Answer from the drawing. Dimensions are ordinates in mm from the lowest x, y and z of the part. Round coordinates to 2 decimals unless told otherwise and drop trailing zeros. Write each loop counter-clockwise with the first axis right and the second up, starting at its lowest first coordinate (ties: lowest second). Pieces come first, ordered by that corner, then holes. Notation, with made-up numbers: (4.25, -37) - (54.25, -37) arc R22 ccw to (54.25, -21) - close; hole circle Ø9 at (22.5, -28.75). An arc over 180 degrees is marked (long way). Answer as a JSON object with one key per item and string values.
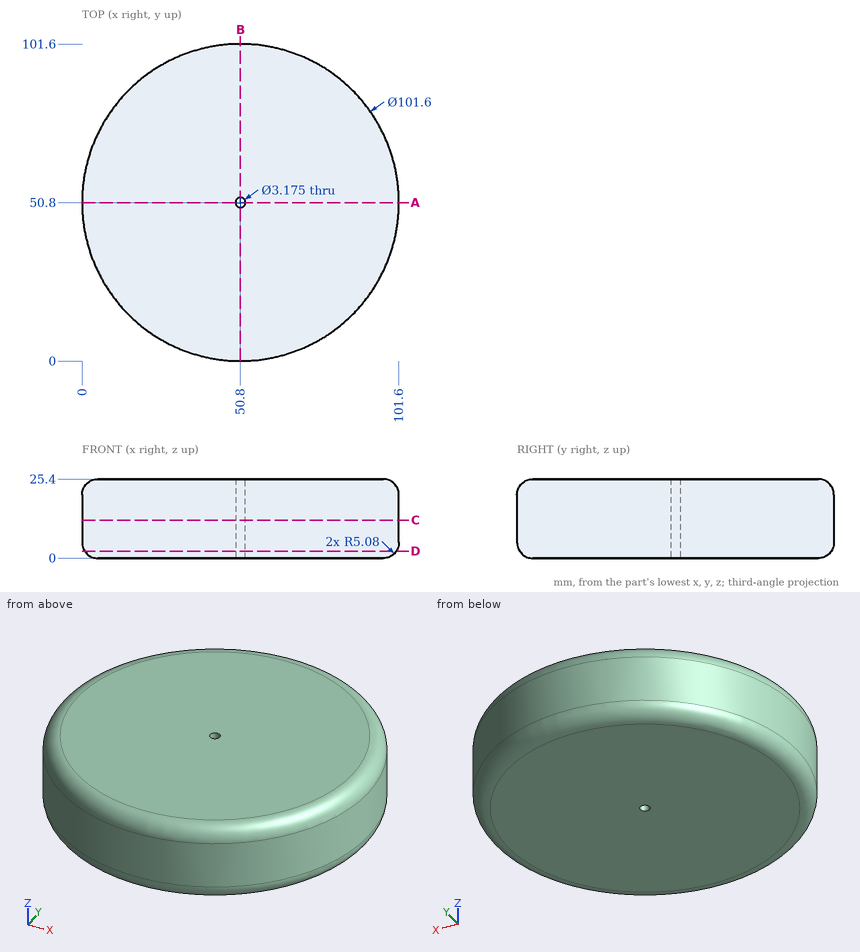
Item 1: A cutting plane is placed at D-D (z = 2.25). Write down the section's boundary in (x, y) (1 decimal), and give its area (3 significant figures).
Results found:
{"outline": "circle Ø99.9 at (50.8, 50.8); hole circle Ø3.2 at (50.8, 50.8)", "area": "7,830 mm²"}
Item 2: Each of these flat-tipped pins is pushed along its axis until it touches: P1, Ø10, axis at y = 21.5, z = 14.5, coming from the +X side; P2, Ø1, axis at x = 73, z = 12, coming from the +Y side; P3, Ø6, axis at x = 71, z = 14, coming from the +Y side; P4, Ø5, axis at x = 42.5, y = 91, coming from the -Z side. Where does it stop, or does it pass through?
Results found:
{"P1": "x = 95.41", "P2": "y = 96.73", "P3": "y = 98.6", "P4": "z = 0"}
Item 3: Consider line 1 along Y through (x, z) = (50.8, 12.25); line 2 along Y through (x, z) = (52, 23); line 3 along Y through (x, z) = (71.5, 12). Determine where each line is inside the solid, lowest interval first.
Results found:
{"line 1": "0 to 49.21, 52.39 to 101.6", "line 2": "0.78 to 49.76, 51.84 to 100.82", "line 3": "4.41 to 97.19"}
Item 4: A cutting plane is placed at C-C (z = 12.25). Write down the section's boundary in (x, y) (1 decimal).
Results found:
{"outline": "circle Ø101.6 at (50.8, 50.8); hole circle Ø3.2 at (50.8, 50.8)"}
Item 5: A cutting plane is placed at A-A (y = 50.8). Write down the section's boundary in (x, z), and give its area (3 significant figures).
Results found:
{"outline": "(0, 5.08) arc R5.08 ccw to (5.08, 0) - (49.21, 0) - (49.21, 25.4) - (5.08, 25.4) arc R5.08 ccw to (0, 20.32) - close; (52.39, 0) - (96.52, 0) arc R5.08 ccw to (101.6, 5.08) - (101.6, 20.32) arc R5.08 ccw to (96.52, 25.4) - (52.39, 25.4) - close", "area": "2,480 mm²"}
